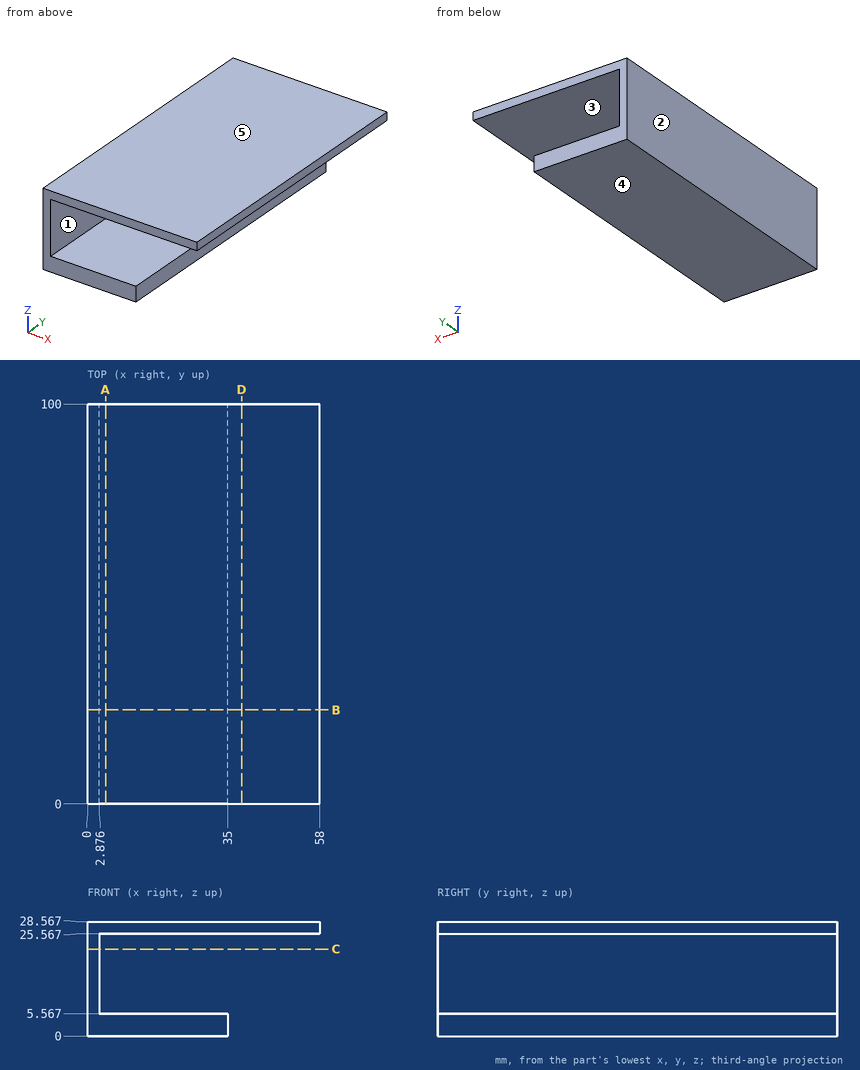
Geometry: see drawing. Coordinates: mm, zero at the bounding-box minimum. A direction names the side the tool comes from. Give positions to 0.01 mm unless a question says otherwise; leave off trailing zeros. Write each loop counter-clockwise with the first axis right and the second up, starting at its lowest first coordinate (ties: lowest second). Pieces come first, ordered by that corner, then holes. Notation, with made-up numbers: M -14,-17.75 L 11,-17.75 A25 ccw 11,-0.75 Z; hole C -2.75,60 d1. An arc over 180 degrees is marked long. Answer in a Markdown table with one row per item. Add a question column.
(1) Ray query, line 1 (Z direction, x = 3, y = 37); line 2 (X direction, y = 75.5, z = 1.5); line 3 (X direction, y = 96.5, z = 23.5). Return the intervals inside material, ascending.
(2) Mould query, pull axis Z, two halves, no side actions, for the marked faces 3, 4 and 5. Classes: +Z half, -Z half, draft (parallel to the pull), parting line (faces both ways), or undercut.
(3) Section B-B on y = 23.5. Return loops of the section in (x, z).
(4) Section D-D on x = 38.5. Return loops of the section in (y, z).
(5) Section A-A on x = 4.5. Return loops of the section in (y, z).
(6) Reachability of the marked faces 1 and 2 from +Z, -Z, +X, -X, +Y, -Y: full face, straight path, thin tool, end or side. Return the list, or none.
(7) First-contact query: pin 1 (4.5 mm diameter, centred on y = 25, z = 2, fed in from +X); pin 2 (10 mm diameter, centred on y = 32.5, z = 13.5, fed in from +X); pin 3 (4 mm diameter, centred on x = 41.5, y = 47, fed in from -Z). Flat tips, straight axial feed; report the tip coordinate or a pass-through.
(8) Section C-C on z = 21.75. Return loops of the section in (x, y), and give its area (3 significant figures).
Result set:
| question | item | result |
|---|---|---|
| 1 | line 1 | z = 0 to 5.57, 25.57 to 28.57 |
| 1 | line 2 | x = 0 to 35 |
| 1 | line 3 | x = 0 to 2.88 |
| 2 | face 3 | undercut |
| 2 | face 4 | -Z half |
| 2 | face 5 | +Z half |
| 3 | outline | M 0,0 L 35,0 L 35,5.57 L 2.88,5.57 L 2.88,25.57 L 58,25.57 L 58,28.57 L 0,28.57 Z |
| 4 | outline | M 0,25.57 L 100,25.57 L 100,28.57 L 0,28.57 Z |
| 5 | outline | M 0,0 L 100,0 L 100,5.57 L 0,5.57 Z; M 0,25.57 L 100,25.57 L 100,28.57 L 0,28.57 Z |
| 6 | face 1 | +X, +Y, -Y |
| 6 | face 2 | +Z, -Z, -X, +Y, -Y |
| 7 | pin 1 | stops at x = 35 |
| 7 | pin 2 | stops at x = 2.88 |
| 7 | pin 3 | stops at z = 25.57 |
| 8 | outline | M 0,0 L 2.88,0 L 2.88,100 L 0,100 Z |
| 8 | area | 288 mm^2 |
